Model file for the job. Use its own axes, mm. Coordinates: 2 decimals unless noted, no trailing zeros. Order: outer loops, then holes, each group sorted by start corner. A loop starts at its lowest first (then second) coordinate and runs counter-clockwise, first axis right, second up. Notation, with made-up numbers: (20.5, 64) -> (78.5, 64) arc R27 cw to (78.5, 89) -> close; hole circle Ø8 at (35, -26). An arc over 180 degrees is marked (long way). Write item = value, one per line. Start each with the question number.
Q1. Flat gauge pins, fed straight in: pin 1 (6 mm diameter, centred on x = 50.5, z = -192.5, fed in from +Y); pin 2 (2 mm diameter, centred on x = 73.5, z = -10.5, fed in from -Y); pin 3 (1.5 mm diameter, centred on y = 1.5, z = -166.5, fed in from -X). Where does each tip first touch, or does it go through?
Q2. Cut at D-D, the plane y = -9.5. List the corners of the cut face in (x, z).
Q3. Wall check: line 1 (X direction, y = 0.85, z = -120); line 2 (Y direction, x = -45, z = -60.5); line 3 (Z direction, x = -5.5, y = 2). Give the ranges that are in metal, low to high. Write a range as from..to.
Q4. Cut at C-C, the plane x = 43.4. List the corners of the cut face in (y, z), plus the area to 3 significant figures.
Q5. Cut at B-B, the plane z = 24.5. List the corners of the cut face in (x, y), plus the area to 3 significant figures.
Q6. Cut at A-A, the plane z = -159. List the corners of the cut face in (x, y), plus the area to 3 significant figures.
from build123d import *

# Parameters (mm, degrees)
SKETCH1_R           = 2
BOSS_EXTRUDE1_DEPTH = 3
SKETCH2_R           = 3
BOSS_EXTRUDE2_DEPTH = 50
SKETCH3_R           = 3.8
BOSS_EXTRUDE3_DEPTH = 30
SKETCH1_3_W         = 25
SKETCH1_3_H         = 40
BOSS_EXTRUDE4_DEPTH = 3
SKETCH4_W           = 5
SKETCH4_H           = 18
CUT_EXTRUDE1_DEPTH  = 10


with BuildPart() as part:
    # Sketch1 → Boss-Extrude1 (new body)
    with BuildSketch(Plane(origin=(0, 0, 0), x_dir=(1, 0, 0), z_dir=(0, 1, 0))):
        with BuildLine():
            ThreePointArc((-100, 25), (-92.67766953, 7.32233047), (-75, 0))
            Line((-75, 0), (-50, 0))
            Line((-50, 0), (50, 0))
            Line((50, 0), (75, 0))
            ThreePointArc((75, 0), (92.67766953, 7.32233047), (100, 25))
            Line((100, 25), (100, 135))
            Line((100, 135), (90, 135))
            Line((90, 135), (90, 200))
            Line((90, 200), (100, 200))
            Line((100, 200), (100, 220))
            Line((100, 220), (-100, 220))
            Line((-100, 220), (-100, 200))
            Line((-100, 200), (-90, 200))
            Line((-90, 200), (-90, 135))
            Line((-90, 135), (-100, 135))
            Line((-100, 135), (-100, 25))
        make_face()
        with BuildLine():
            Line((-14, 45), (-14, 75))
            ThreePointArc((-14, 75), (-12.5, 76.5), (-11, 75))
            Line((-11, 75), (-11, 45))
            ThreePointArc((-11, 45), (-12.5, 43.5), (-14, 45))
        make_face(mode=Mode.SUBTRACT)
        with BuildLine():
            ThreePointArc((11, 75), (12.5, 76.5), (14, 75))
            Line((14, 75), (14, 45))
            ThreePointArc((14, 45), (12.5, 43.5), (11, 45))
            Line((11, 45), (11, 75))
        make_face(mode=Mode.SUBTRACT)
        with Locations(Location((-90, 110, 0), (0, 0, 270))):
            Circle(SKETCH1_R, mode=Mode.SUBTRACT)
        with Locations(Location((-90, 120, 0), (0, 0, 270))):
            Circle(SKETCH1_R, mode=Mode.SUBTRACT)
        with BuildLine():
            Line((-14, 150), (-14, 180))
            ThreePointArc((-14, 180), (-12.5, 181.5), (-11, 180))
            Line((-11, 180), (-11, 150))
            ThreePointArc((-11, 150), (-12.5, 148.5), (-14, 150))
        make_face(mode=Mode.SUBTRACT)
        with BuildLine():
            Line((-62.5, 211.5), (-12.5, 211.5))
            ThreePointArc((-12.5, 211.5), (-11, 210), (-12.5, 208.5))
            Line((-12.5, 208.5), (-62.5, 208.5))
            ThreePointArc((-62.5, 208.5), (-64, 210), (-62.5, 211.5))
        make_face(mode=Mode.SUBTRACT)
        with Locations(Location((90, 110, 0), (0, 0, 270))):
            Circle(SKETCH1_R, mode=Mode.SUBTRACT)
        with Locations(Location((90, 120, 0), (0, 0, 270))):
            Circle(SKETCH1_R, mode=Mode.SUBTRACT)
        with BuildLine():
            ThreePointArc((11, 180), (12.5, 181.5), (14, 180))
            Line((14, 180), (14, 150))
            ThreePointArc((14, 150), (12.5, 148.5), (11, 150))
            Line((11, 150), (11, 180))
        make_face(mode=Mode.SUBTRACT)
        with BuildLine():
            ThreePointArc((12.5, 208.5), (11, 210), (12.5, 211.5))
            Line((12.5, 211.5), (62.5, 211.5))
            ThreePointArc((62.5, 211.5), (64, 210), (62.5, 208.5))
            Line((62.5, 208.5), (12.5, 208.5))
        make_face(mode=Mode.SUBTRACT)
    extrude(amount=BOSS_EXTRUDE1_DEPTH)

    # Sketch2 → Boss-Extrude2 (add)
    with BuildSketch(Plane(origin=(0, 3, 0), x_dir=(1, 0, 0), z_dir=(0, 1, 0))):
        with Locations(Location((-80, 20, 0), (0, 0, 270))):
            Circle(SKETCH2_R)
        with Locations(Location((80, 20, 0), (0, 0, 270))):
            Circle(SKETCH2_R)
        with Locations(Location((-80, 180, 0), (0, 0, 270))):
            Circle(SKETCH2_R)
        with Locations(Location((80, 180, 0), (0, 0, 270))):
            Circle(SKETCH2_R)
    extrude(amount=BOSS_EXTRUDE2_DEPTH)

    # Sketch3 → Boss-Extrude3 (add)
    with BuildSketch(Plane(origin=(0, 0, 0), x_dir=(1, 0, 0), z_dir=(0, 1, 0))):
        with Locations(Location((-43.4, 50, 0), (0, 0, 270))):
            Circle(SKETCH3_R)
        with Locations(Location((43.4, 50, 0), (0, 0, 270))):
            Circle(SKETCH3_R)
    extrude(amount=-BOSS_EXTRUDE3_DEPTH)

    # Sketch1_3 → Boss-Extrude4 (add)
    with BuildSketch(Plane(origin=(0, 0, 0), x_dir=(1, 0, 0), z_dir=(0, 1, 0))):
        with Locations((-62.5, -20)):
            Rectangle(SKETCH1_3_W, SKETCH1_3_H)
        with Locations((62.5, -20)):
            Rectangle(SKETCH1_3_W, SKETCH1_3_H)
    extrude(amount=BOSS_EXTRUDE4_DEPTH)

    # Sketch4 → Cut-Extrude1 (cut)
    with BuildSketch(Plane(origin=(0, 3, 0), x_dir=(1, 0, 0), z_dir=(0, 1, 0))):
        with Locations((-52.5, -26)):
            Rectangle(SKETCH4_W, SKETCH4_H)
        with Locations((52.5, -26)):
            Rectangle(SKETCH4_W, SKETCH4_H)
    extrude(amount=-CUT_EXTRUDE1_DEPTH, mode=Mode.SUBTRACT)


solid = part.part
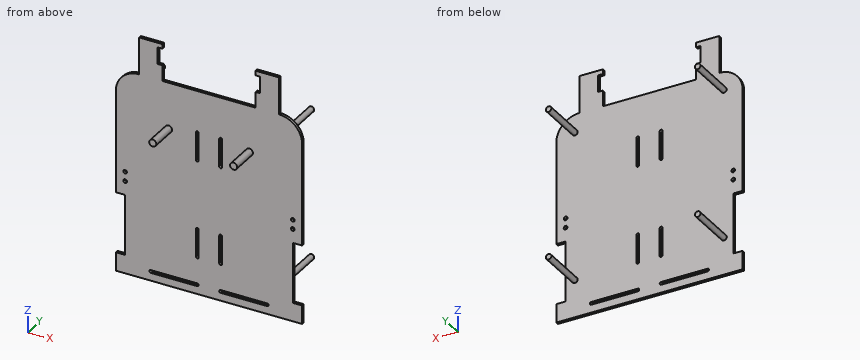
Here are the results:
q1.pin_1 = 3
q1.pin_2 = 0
q1.pin_3 = -90
q2.outline = circle Ø7.6 at (-43.4, -50); circle Ø7.6 at (43.4, -50)
q3.line_1 = -100..-92, -88..88, 92..100
q3.line_2 = 0..3
q3.line_3 = -220..0
q4.outline = (-30, -53.8) -> (0, -53.8) -> (0, -208.5) -> (3, -208.5) -> (3, 0) -> (0, 0) -> (0, -46.2) -> (-30, -46.2) -> close; (0, -220) -> (3, -220) -> (3, -211.5) -> (0, -211.5) -> close
q4.area = 879 mm²
q5.outline = (-75, 0) -> (-55, 0) -> (-55, 3) -> (-75, 3) -> close; (55, 0) -> (75, 0) -> (75, 3) -> (55, 3) -> close
q5.area = 120 mm²
q6.outline = (-90, 0) -> (-14, 0) -> (-14, 3) -> (-90, 3) -> close; (-11, 0) -> (11, 0) -> (11, 3) -> (-11, 3) -> close; (14, 0) -> (90, 0) -> (90, 3) -> (14, 3) -> close
q6.area = 522 mm²
